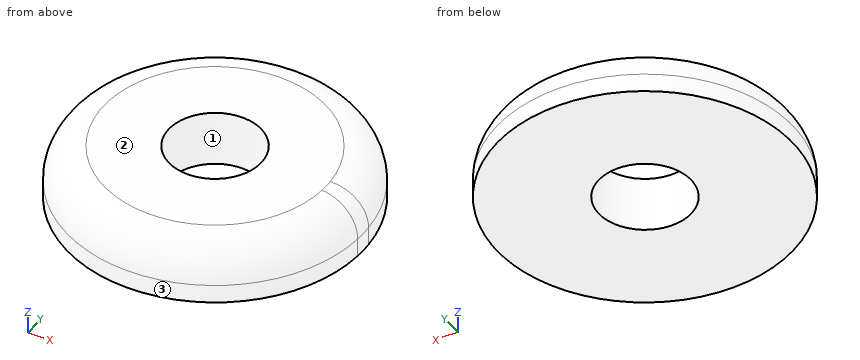
Autodesk Inventor part; units mm, degrees
ref_plane "YZ Plane" through (0, 0, 0) normal (1, 0, 0) x (0, 1, 0)
ref_plane "XZ Plane" through (0, 0, 0) normal (0, 1, 0) x (-1, 0, 0)
ref_plane "XY Plane" through (0, 0, 0) normal (0, 0, 1) x (1, 0, 0)
sketch "Эскиз1" plane through (0, 0, 0) normal (0, 0, 1) x (1, 0, 0)
  line L0 (-4.0768, 1.9994) -> (-0.6127, 3.9994)
  line L1 (-0.6127, 3.9994) -> (2.8514, 1.9994)
  line L2 (2.8514, 1.9994) -> (2.8353, 0.4994)
  line L3 (2.8353, 0.4994) -> (7.3716, 0.4994)
  arc A0 (7.3716, 0.4994) -> (7.3716, -0.5006) centre (-0.6127, -0.0006) ccw
  line L4 (7.3716, -0.5006) -> (2.8246, -0.5006)
  line L5 (2.8246, -0.5006) -> (2.8082, -2.0255)
  line L6 (2.8082, -2.0255) -> (-0.6127, -4.0006)
  line L7 (-0.6127, -4.0006) -> (-4.0768, -2.0006)
  line L8 (-4.0768, -2.0006) -> (-4.0768, 1.9994)
  circle A1 centre (-0.6127, -0.0006) radius 8
  point P0 (0, 0)
extrude "Выдавливание1" add sketch "Эскиз1" along normal blind 3
fillet "Сопряжение1" radius 2 1 edges at (-8.6127, -0.0006, 3)
sketch "Эскиз2" plane through (-0.6127, -0.0006, 3) normal (0, 0, 1) x (1, 0, 0)
  circle A0 centre (0, 0) radius 2.5
  point P0 (0.6127, 0.0006)
  dimension "d3" = 5
extrude "Выдавливание2" cut sketch "Эскиз2" against normal blind 3
properties part number "SecindaryCap"
Source: CAD feature listing. Evaluate the final solid. Frame: model axes, mm. Face numbers are marked on the shaded views. Round coordinates to 2 decimals unless told otherwise and drop trailing zeros. Loops run counter-clockwise (first coordinate to the right, second up) from the corner with the lowest first, then second, coordinate; pieces in that order, holes last. Notation, with made-up numbers: (47, 30.25) -> (83, 30.25) arc R31 ccw to (83, 56.25) -> close; hole circle Ø9 at (9, 65.25). An arc over 180 degrees is marked (long way). Answer as a JSON object with one key per item and string values. Group by question number.
Q1. Mould query, pull axis X, two halves, no side actions, for the marked faces 1, 2 and 3. Classes: pulls with the +X half, pulls with the -X half, needs draft (parallel to the pull), parting line crosses it, or undercut.
Q2. Section query B-B (z = 2). Output: boundary loops of the cut face in (x, y).
Q3. Section query A-A (z = 0.5). Output: boundary loops of the cut face in (x, y), plus the area to 3 significant figures.
Q4. Contact query for flat-ended pins moving along their axis: P1, Ø1, axis at x = 1, z = 1, coming from the -Y side; P2, Ø4.5, axis at x = -0.61, y = 0, coming from the -Z side. Output: stop coordinate, or through.
Q5. Ray query, line 1 (Y direction, x = -0.5, z = 1.2); line 2 (X direction, y = 2, z = 2.5); line 3 (Y direction, x = -1.25, z = 1.8). Return the intervals inside material, ascending. Write a range as from..to.
Completed:
{
 "1": {"face 1": "undercut", "face 2": "needs draft", "face 3": "parting line crosses it"},
 "2": {"outline": "(7.1, -0.48) arc R7.73 ccw to (7.1, 0.48) arc R7.73 ccw (long way) to start; hole circle Ø5 at (-0.61, 0)"},
 "3": {"outline": "circle Ø16 at (-0.61, 0); hole circle Ø5 at (-0.61, 0)", "area": "181 mm²"},
 "4": {"P1": "y = -7.92", "P2": "through"},
 "5": {"line 1": "-7.99..-2.5, 2.5..7.99", "line 2": "-7.66..-2.11, 0.89..6.43", "line 3": "-7.81..-2.42, 2.42..7.81"}
}
